Can you work these out from the model? Positions are in its coordinate system, mm. Face numbers are marked on the shaded views. A direction names the side the tool comes from. Round coordinates to 2 decimals unless told otherwise and drop trailing zeros. Loops run counter-clockwise (first coordinate to the right, second up) from the corner with the lowest first, then second, coordinate; pieces in that order, holes last.
(1) I want a section at A-A on x = 0. Write out the boundary of the cut face in (y, z), plus the area to 3 significant figures.
(2) I want a section at B-B on y = 0. Write out the boundary of the cut face in (x, z).
(3) Thinking about a two-plate mould opening in Y: for the marked faces 3, 4 and 5, which applies, released by +Y, released by -Y, zero draft, split by the parting line, or undercut?
(4) Which directions (+Z, -Z, +X, -X, +Y, -Y) give clear straight access to the entire face, cutting with the end or side of a thin tool? Please do the marked faces 1 and 2.
(5) I want a section at C-C on z = 0.8. Write out the boundary of the cut face in (x, y).
(6) I want a section at D-D on x = -1.75. Write out the boundary of the cut face in (y, z).
(7) Will these pins go through, and if not, where does the flat tip stop? pin 1 Ø5 at (x, y) = (-3, 0) entering from -Z; pin 2 Ø0.6 at (y, z) = (4, 2) entering from -X; pin 3 Ø0.6 at (x, z) = (0.5, 2) entering from +Y; pin 4 Ø0.9 at (y, z) = (3.5, 2) entering from +X.
(8) If I drill on line 1 along Y through (x, z) = (0, 2.95); line 2 along Z through (x, y) = (3.75, 1); line 3 along Y through (x, z) = (1, 2.1), over which ranges is the centre line in solid material (lowest first)?
from build123d import *

# Parameters (mm, degrees)
SKETCH1_R           = 7
BOSS_EXTRUDE1_DEPTH = 1.5
SKETCH2_W           = 5.5
SKETCH2_H           = 5
BOSS_EXTRUDE2_DEPTH = 1.5
SKETCH3_R           = 2
CUT_EXTRUDE1_DEPTH  = 0.2
SKETCH4_W           = 1.6
SKETCH4_H           = 0.8
BOSS_EXTRUDE3_DEPTH = 0.8


with BuildPart() as part:
    # Sketch1 → Boss-Extrude1 (new body)
    with BuildSketch(Plane.XY):
        Circle(SKETCH1_R)
    extrude(amount=BOSS_EXTRUDE1_DEPTH)

    # Sketch2 → Boss-Extrude2 (add)
    with BuildSketch(Plane.XY.offset(1.5)):
        Rectangle(SKETCH2_W, SKETCH2_H)
    extrude(amount=BOSS_EXTRUDE2_DEPTH)

    # Sketch3 → Cut-Extrude1 (cut)
    with BuildSketch(Plane.XY.offset(3)):
        Circle(SKETCH3_R)
    extrude(amount=-CUT_EXTRUDE1_DEPTH, mode=Mode.SUBTRACT)

    # Sketch4 → Boss-Extrude3 (add)
    with BuildSketch(Plane.XY.offset(1.5)):
        with Locations((0, 3.7)):
            Rectangle(SKETCH4_W, SKETCH4_H)
    extrude(amount=BOSS_EXTRUDE3_DEPTH)


solid = part.part
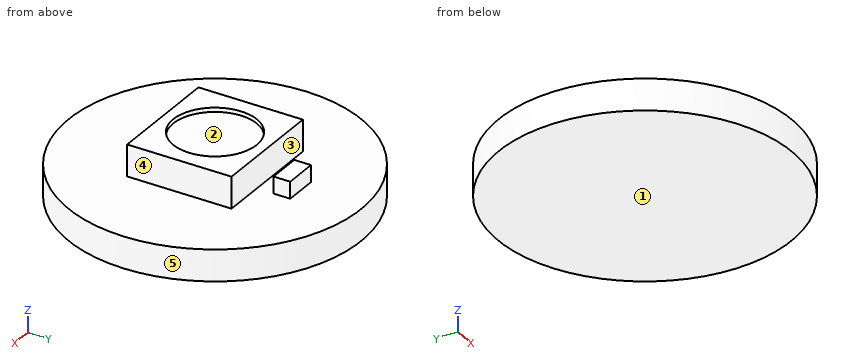
Filled sheet:
1. outline: (-7, 0) - (7, 0) - (7, 1.5) - (4.1, 1.5) - (4.1, 2.3) - (3.3, 2.3) - (3.3, 1.5) - (2.5, 1.5) - (2.5, 3) - (2, 3) - (2, 2.8) - (-2, 2.8) - (-2, 3) - (-2.5, 3) - (-2.5, 1.5) - (-7, 1.5) - close
1. area: 28.3 mm2
2. outline: (-7, 0) - (7, 0) - (7, 1.5) - (2.75, 1.5) - (2.75, 3) - (2, 3) - (2, 2.8) - (-2, 2.8) - (-2, 3) - (-2.75, 3) - (-2.75, 1.5) - (-7, 1.5) - close
3. face 3: undercut
3. face 4: zero draft
3. face 5: split by the parting line
4. face 1: -Z, +X, -X, +Y, -Y
4. face 2: +Z
5. outline: circle Ø14 at (0, 0)
6. outline: (-6.78, 0) - (6.78, 0) - (6.78, 1.5) - (2.5, 1.5) - (2.5, 3) - (0.97, 3) - (0.97, 2.8) - (-0.97, 2.8) - (-0.97, 3) - (-2.5, 3) - (-2.5, 1.5) - (-6.78, 1.5) - close
7. pin 1: stops at z = 0
7. pin 2: stops at x = -0.8
7. pin 3: stops at y = 4.1
7. pin 4: stops at x = 0.8
8. line 1: y = -2.5 to -2, 2 to 2.5
8. line 2: z = 0 to 1.5
8. line 3: y = -2.5 to 2.5
